Could you check a few things on this model? Use its own coordinates, in mm. A direction names the side the tool comes from. Give positions to 0.01 mm unless a question says otherwise; leave off trailing zeros. Loops run counter-clockwise (first coordinate to the right, second up) from the corner with the lowest first, then second, coordinate; pieces in that order, holes last. Notation, with made-up numbers: M 77,83.25 L 119,83.25 A19 cw 119,111.25 Z; hole C 35,37 d3. An arc over 180 degrees is marked long. Write each question's results on one line, items separated by ' | '. Start each with the question number.
from build123d import *

# Parameters (mm, degrees)
EXTRUDE_1_DEPTH = 200


with BuildPart() as part:
    # 草图2 → 凸台-拉伸1 (new body)
    with BuildSketch(Plane.XY):
        with BuildLine():
            Line((0, 10), (0, 115))
            ThreePointArc((0, 115), (2.928932188, 122.071067812), (10, 125))
            Line((10, 125), (90, 125))
            Line((90, 125), (100, 125))
            Line((100, 125), (100, 130))
            Line((100, 130), (10, 130))
            ThreePointArc((10, 130), (-0.606601718, 125.606601718), (-5, 115))
            Line((-5, 115), (-5, 20))
            Line((-5, 20), (-5, 10))
            Line((-5, 10), (0, 10))
        make_face()
    extrude(amount=EXTRUDE_1_DEPTH)


solid = part.part
1) If we section it at B-B on y = 110: Write out the boundary of the cut face in (x, z), plus the area to 3 significant figures.
2) If we section it at C-C on x = 58.5: Write out the boundary of the cut face in (y, z), plus the area to 3 significant figures.
3) I'm going to push a flat-ended pin straight in: P1, Ø5, axis at x = 34.5, z = 35.5, coming from the -Y side. Where does the tip first touch, or does it pass through?
4) Which directions (+Z, -Z, +X, -X, +Y, -Y) give clear straight access to the entire face, cutting with the end or side of a thin tool? Please do faces 1 (the face through (54, 125, 99)), 2 (the face through (-0.49, 125.72, 98.6)).
5) Please list where these lines run through material, in increasing order: line 1 (X direction, y = 79.5, z = 28); line 2 (Y direction, x = 27, z = 116); line 3 (Y direction, x = 5, z = 69.5). Write a range as from..to.
6) If we section it at A-A on z = 53: Write out the boundary of the cut face in (x, y).
Calculated:
1) outline: M -5,0 L 0,0 L 0,200 L -5,200 Z | area: 1,000 mm2
2) outline: M 125,0 L 130,0 L 130,200 L 125,200 Z | area: 1,000 mm2
3) P1: stops at y = 125
4) face 1: +Z, -Z, +X, -Y | face 2: +Z, -Z, -X, +Y
5) line 1: x = -5..0 | line 2: y = 125..130 | line 3: y = 123.66..129.14
6) outline: M -5,10 L 0,10 L 0,115 A10 cw 10,125 L 100,125 L 100,130 L 10,130 A15 ccw -5,115 Z
